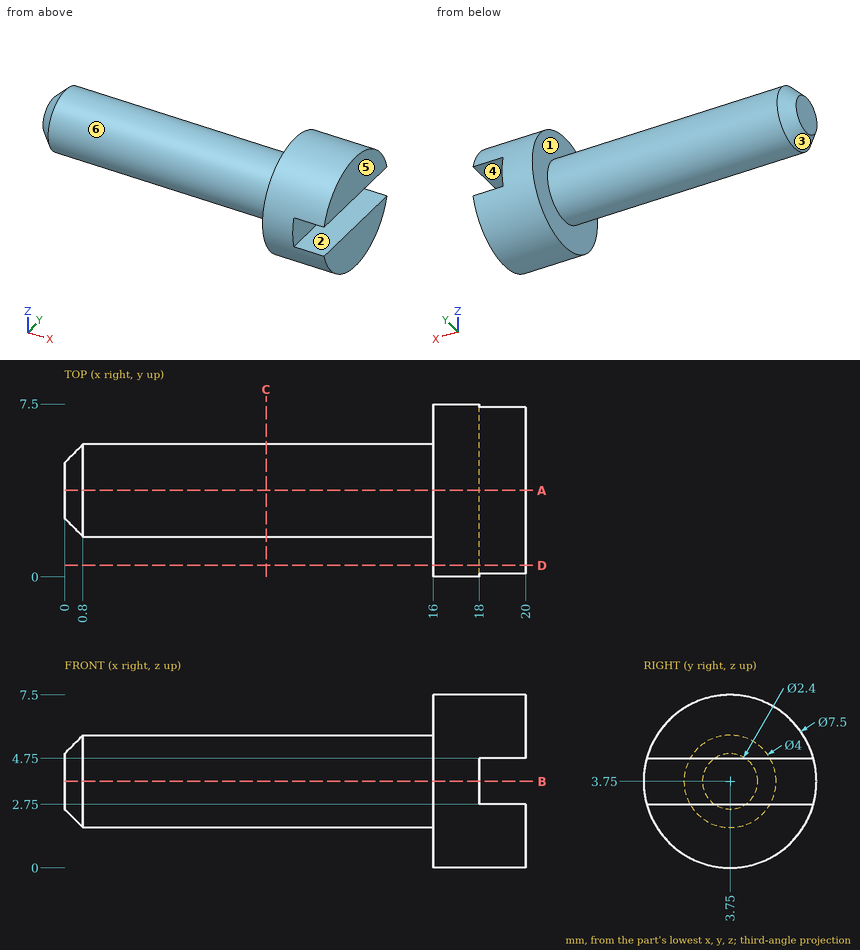
Study the drawing (mm; zero at the part's minimum x, y, z) and answer. A direction names the side the tool comes from. Give positions to 0.01 mm unless a question says otherwise; leave off trailing zeros. Write each loop counter-clockwise with the first axis right and the second up, starting at its lowest first coordinate (ties: lowest second). Pieces come first, ordered by that corner, then holes. Notation, with made-up numbers: (3, -28.75) -> (39, -28.75) arc R18 ccw to (39, -7.75) -> close; hole circle Ø9 at (22, -39). An arc over 180 degrees is marked (long way). Write item = value, one per line.
Q1. Section C-C on x = 8.75 is taken. Determine the outline of the cut face in (y, z), and give its area (3 significant figures).
Computed values:
outline = circle Ø4 at (3.75, 3.75)
area = 12.6 mm^2
Q2. For a pull along Z with two mould halves and no side action, classify the marked faces 1, 2 and 3 as pulls with the +Z half, pulls with the -Z half, needs draft (parallel to the pull), parting line crosses it, or undercut.
Computed values:
face_1 = needs draft
face_2 = undercut
face_3 = parting line crosses it
Q3. Consider line 1 along X through (y, z) = (6.5, 4.5); line 2 along X through (y, z) = (1.5, 2); line 3 along Y through (x, z) = (16.5, 5.5). Determine where each line is inside the solid, lowest interval first.
Computed values:
line_1 = 16 to 18
line_2 = 16 to 20
line_3 = 0.43 to 7.07
Q4. Section D-D on y = 0.5 is taken. Determine the outline of the cut face in (x, z), and give its area (3 significant figures).
Computed values:
outline = (16, 1.88) -> (20, 1.88) -> (20, 2.75) -> (18, 2.75) -> (18, 4.75) -> (20, 4.75) -> (20, 5.62) -> (16, 5.62) -> close
area = 11.0 mm^2
Q5. Section A-A on y = 3.75 is taken. Determine the outline of the cut face in (x, z), and give its area (3 significant figures).
Computed values:
outline = (0, 2.55) -> (0.8, 1.75) -> (16, 1.75) -> (16, 0) -> (20, 0) -> (20, 2.75) -> (18, 2.75) -> (18, 4.75) -> (20, 4.75) -> (20, 7.5) -> (16, 7.5) -> (16, 5.75) -> (0.8, 5.75) -> (0, 4.95) -> close
area = 89.4 mm^2
Q6. Section B-B on z = 3.75 is taken. Determine the outline of the cut face in (x, y).
Computed values:
outline = (0, 2.55) -> (0.8, 1.75) -> (16, 1.75) -> (16, 0) -> (18, 0) -> (18, 7.5) -> (16, 7.5) -> (16, 5.75) -> (0.8, 5.75) -> (0, 4.95) -> close
Q7. Flat-ended cylindrical pins translate along their axes: pin 1 Ø0.6 at (x, y) = (19, 5) entering from -Z; pin 2 Ø1 at (x, y) = (10.5, 3.5) entering from +Z; pin 3 Ø1 at (x, y) = (18.5, 5) entering from +Z. Find the tip coordinate at first contact, or state that the pin passes through.
Computed values:
pin_1 = 0.12
pin_2 = 5.75
pin_3 = 7.42
Q8. A tool of negligible diameter and unlimited length cuts with its end or side. For the marked faces 4, 5 and 6, from which of +Z, -Z, +X, -X, +Y, -Y can it reach the whole face along a straight path? Write none if from no direction.
Computed values:
face_4 = +X, +Y, -Y
face_5 = +Z, -Z, +X, +Y, -Y
face_6 = -X
